CAD build for the part. Positions are in the model's coordinates, mm. A direction names the side the tool comes from. Coordinates: 2 decimals unless noted, no trailing zeros. Order: outer loops, then holes, each group sorted by start corner. A loop starts at its lowest first (then second) coordinate and runs counter-clockwise, first axis right, second up. Notation, with made-up numbers: M 13,18 L 29,18 A24 ccw 29,43 Z; hole C -14.5,55 d1. An arc over 180 degrees is marked long. Write item = value, one per line.
from build123d import *

# Parameters (mm, degrees)
SKETCH1_R           = 1.75
SKETCH1_W           = 5
SKETCH1_H           = 5
BOSS_EXTRUDE1_DEPTH = 5


with BuildPart() as part:
    # Sketch1 → Boss-Extrude1 (new body)
    with BuildSketch(Plane.XY):
        with BuildLine():
            Line((0, 10), (32.5, 10))
            Line((32.5, 10), (32.5, -10))
            Line((32.5, -10), (0, -10))
            ThreePointArc((0, -10), (-10, 0), (0, 10))
        make_face()
        Circle(SKETCH1_R, mode=Mode.SUBTRACT)
        with Locations((27.5, 5)):
            Rectangle(SKETCH1_W, SKETCH1_H, mode=Mode.SUBTRACT)
        with Locations((27.5, -5)):
            Rectangle(SKETCH1_W, SKETCH1_H, mode=Mode.SUBTRACT)
        with Locations((20, -5)):
            Rectangle(SKETCH1_W, SKETCH1_H, mode=Mode.SUBTRACT)
        with Locations((20, 5)):
            Rectangle(SKETCH1_W, SKETCH1_H, mode=Mode.SUBTRACT)
    extrude(amount=BOSS_EXTRUDE1_DEPTH)


solid = part.part
(1) Slice it at D-D, the plane x = -6. Write the cut outline in (y, z), then the cut area to 3 significant figures.
Evaluation:
outline = M -8,0 L 8,0 L 8,5 L -8,5 Z
area = 80.0 mm²
(2) Slice it at B-B, the plane y = 0. Write the cut outline in (x, z).
Evaluation:
outline = M -10,0 L -1.75,0 L -1.75,5 L -10,5 Z; M 1.75,0 L 32.5,0 L 32.5,5 L 1.75,5 Z
(3) Slice it at A-A, the plane z = 3.8. Write the cut outline in (x, y).
Evaluation:
outline = M 0,-10 L 32.5,-10 L 32.5,10 L 0,10 A10 ccw Z; hole C 0,0 d3.5; hole M 17.5,-7.5 L 22.5,-7.5 L 22.5,-2.5 L 17.5,-2.5 Z; hole M 17.5,2.5 L 22.5,2.5 L 22.5,7.5 L 17.5,7.5 Z; hole M 25,-7.5 L 30,-7.5 L 30,-2.5 L 25,-2.5 Z; hole M 25,2.5 L 30,2.5 L 30,7.5 L 25,7.5 Z
(4) Pull direction Y, two halves, no side cores. Call faces 1 (the face through (25, -5, 2)), 2 (the face through (-10, 0, 2)), 3 (the face through (12, 0, 5)): +Y half, -Y half, draft (parallel to the pull), parting line (faces both ways), or undercut.
Evaluation:
face_1 = undercut
face_2 = parting line
face_3 = draft
(5) Slice it at C-C, the plane y = -5.25. Write the cut outline in (x, z).
Evaluation:
outline = M -8.51,0 L 17.5,0 L 17.5,5 L -8.51,5 Z; M 22.5,0 L 25,0 L 25,5 L 22.5,5 Z; M 30,0 L 32.5,0 L 32.5,5 L 30,5 Z
(6) Tool access for faces 4 (the face through (27, -2.5, 2)), 5 (the face through (32.5, 0, 2)): list every direction of +Z, -Z, +X, -X, +Y, -Y with a clear straight run to the whole face (end or side of a thin tool).
Evaluation:
face_4 = +Z, -Z
face_5 = +Z, -Z, +X, +Y, -Y
(7) Pin check, flat tips, straight feed: pin 1 Ø1.5 at (y, z) = (5, 1.5) entering from -X; pin 2 Ø3 at (x, y) = (0, 0) entering from +Z; pin 3 Ø2 at (y, z) = (-2.5, 2.5) entering from -X; pin 4 Ø1.5 at (y, z) = (-5.5, 2.5) entering from -X. Stop position of each tip, or through.
Evaluation:
pin_1 = -9.05
pin_2 = through
pin_3 = -9.89
pin_4 = -8.8
(8) Wall check: line 1 (Y direction, x = 21, z = 1.7); line 2 (Y direction, x = 0, z = 1.25); line 3 (X direction, y = -7, z = 1.1). Give the ranges that are in metal, low to high. Write a range as from..to.
Evaluation:
line_1 = -10..-7.5, -2.5..2.5, 7.5..10
line_2 = -10..-1.75, 1.75..10
line_3 = -7.14..17.5, 22.5..25, 30..32.5
